from build123d import *

# Parameters (mm, degrees)
PAD_DEPTH       = 7
SKETCH001_R     = 2.75
POCKET_DEPTH    = 37.501
SKETCH002_R     = 3.5
POCKET001_DEPTH = 5
SKETCH003_R     = 1.5
POCKET002_DEPTH = 26.001
FILLET_R        = 0.5
CHAMFER_SIZE    = 0.75
CHAMFER001_SIZE = 0.75
CHAMFER002_SIZE = 0.75
CHAMFER003_SIZE = 0.5


with BuildPart() as part:
    # Sketch → Pad (new body, symmetric)
    with BuildSketch(Plane.XZ):
        with BuildLine():
            Line((-21, 0), (21, 0))
            Line((21, 0), (21, 6))
            Line((21, 6), (10, 6))
            Line((10, 6), (10, 37.5))
            Line((10, 37.5), (1, 37.5))
            Line((1, 37.5), (1, 28.91608))
            ThreePointArc((-1, 28.91608), (0, 17), (1, 28.91608))
            Line((-1, 37.5), (-1, 28.91608))
            Line((-1, 37.5), (-10, 37.5))
            Line((-10, 37.5), (-10, 6))
            Line((-10, 6), (-21, 6))
            Line((-21, 6), (-21, 0))
        make_face()
    extrude(amount=PAD_DEPTH, both=True)

    # Sketch001 → Pocket (cut, through all)
    with BuildSketch(Plane(origin=(0, 0, 0), x_dir=(1, 0, 0), z_dir=(0, 0, -1))):
        with Locations((16, 0)):
            Circle(SKETCH001_R)
        with Locations((-16, 0)):
            Circle(SKETCH001_R)
    extrude(amount=-POCKET_DEPTH, mode=Mode.SUBTRACT)

    # Sketch002 → Pocket001 (cut)
    with BuildSketch(Plane(origin=(10, 0, 0), x_dir=(0, 0, 1), z_dir=(1, 0, 0))):
        with Locations((32, 0)):
            Circle(SKETCH002_R)
    extrude(amount=-POCKET001_DEPTH, mode=Mode.SUBTRACT)

    # Sketch003 → Pocket002 (cut, through all)
    with BuildSketch(Plane(origin=(5, 0, 0), x_dir=(0, 0, 1), z_dir=(1, 0, 0))):
        with Locations((32, 0)):
            Circle(SKETCH003_R)
    extrude(amount=-POCKET002_DEPTH, mode=Mode.SUBTRACT)

    # Fillet
    fillet_edges = [part.edges().sort_by_distance(p)[0] for p in [
        (21, 0, 6),
        (10, 0, 6),
        (10, 0, 37.5),
        (-10, 0, 37.5),
        (-10, 0, 6),
        (-21, 0, 6),
    ]]
    fillet(fillet_edges, radius=FILLET_R)

    # Chamfer
    chamfer_edges = [part.edges().sort_by_distance(p)[0] for p in [
        (13.25, 0, 6),
        (-18.75, 0, 6),
    ]]
    chamfer(chamfer_edges, length=CHAMFER_SIZE)

    # Chamfer001
    chamfer001_edges = [part.edges().sort_by_distance(p)[0] for p in [
        (10, 0, 28.5),
    ]]
    chamfer(chamfer001_edges, length=CHAMFER001_SIZE)

    # Chamfer002
    chamfer002_edges = [part.edges().sort_by_distance(p)[0] for p in [
        (-10, 0, 30.5),
    ]]
    chamfer(chamfer002_edges, length=CHAMFER002_SIZE)

    # Chamfer003
    chamfer003_edges = [part.edges().sort_by_distance(p)[0] for p in [
        (0, 7, 17),
        (0, -7, 17),
    ]]
    chamfer(chamfer003_edges, length=CHAMFER003_SIZE)


solid = part.part
Design review of the part built by this model. Coordinates are the model's own, in mm. A direction names the side the tool comes from. Give positions to 0.01 mm unless a question says otherwise; leave off trailing zeros. Loops run counter-clockwise (first coordinate to the right, second up) from the corner with the lowest first, then second, coordinate; pieces in that order, holes last. Notation, with made-up numbers: M 3,49.5 L 26,49.5 A21 ccw 26,66.5 Z; hole C 42,7 d3. An arc over 180 degrees is marked long. One line per question, with ' | ' between items. Start each with the question number.
1. Add section A-A (x = -16). Write out the cut boundary in (y, z), plus the area to 3 significant figures.
2. For faces 1 (the face through (3.03, -0.07, 30.5)), 2 (the face through (-12, 0, 6)), 3 (the face through (12, 0, 6)), list the 3-axis set-ups (+Z, -Z, +X, -X, +Y, -Y) from which the entire face can be reached by the end or side of a thin tool; tool diameter is ignored.
3. Add section D-D (x = 0). Write out the cut boundary in (y, z).
4. Insertion check: P1, Ø2.5, axis at y = 0, z = 32, coming from the +X side; P2, Ø5, axis at x = -17, y = 3, coming from the +Z side; P3, Ø4, axis at y = -2.5, z = 16, coming from the +X side; P4, Ø3.5, axis at y = 0, z = 33, coming from the +X side. Each pin has a flat end and moves straight along its axis. Give the tip position at first contact, or say it passes through.
5. The part is to be moulded in two halves that separate along X. For faces 4 (the face through (-18.747, -0.121, 2.588)), 5 (the face through (10, 0, 22)), 6 (the face through (0, -7, 15)), say which applies: released by +X, released by -X, zero draft, split by the parting line, or undercut.
6. Add section C-C (y = 0). Give the number of separate pieces and of enclosed holes in the cut face, plus the area to 3 significant figures.
7. To check wall thickness, follow L1, parallel to Z at x = -7.5, y = 0; L2, parallel to Y at x = -5, z = 32; L3, parallel to X at y = 1.25, z = 29. State the ranges of each line that lie inside material, in increasing order.
8. Add section B-B (z = 23). Write out the cut boundary in (x, y), plus the area to 4 significant figures.
Worked out:
1) outline: M -7,0 L -2.75,0 L -2.75,5.25 L -3.5,6 L -7,6 Z; M 2.75,0 L 7,0 L 7,6 L 3.5,6 L 2.75,5.25 Z | area: 50.4 mm²
2) face 1: +X, -X | face 2: +Z, -X, +Y, -Y | face 3: +Z, +X, +Y, -Y
3) outline: M -7,0 L 7,0 L 7,16.5 L 6.5,17 L -6.5,17 L -7,16.5 Z
4) P1: passes through | P2: stops at z = 6 | P3: stops at x = 10 | P4: stops at x = 5
5) face 4: undercut | face 5: released by +X | face 6: zero draft
6) separate pieces: 5 | enclosed holes: 0 | area: 609 mm²
7) L1: z = 0 to 30.5, 33.5 to 37.5 | L2: y = -7 to -1.5, 1.5 to 7 | L3: x = -10 to -1, 1 to 5
8) outline: M -10,-7 L -6.5,-7 L -6,-6.5 L -6,6.5 L -6.5,7 L -10,7 Z; M 6,-6.5 L 6.5,-7 L 10,-7 L 10,7 L 6.5,7 L 6,6.5 Z | area: 111.5 mm²
